Could you check a few things on this model? Use its own coordinates, in mm. A direction names the side the tool comes from. Coordinates: 2 decimals unless noted, no trailing zeros. Write each loop counter-clockwise with the first axis right and the second up, starting at its lowest first coordinate (ties: lowest second). Pieces come first, ordered by that corner, then holes. Notation, with made-up numbers: M 51,67.5 L 110,67.5 A14 cw 110,76.5 Z; hole C 2,17 d4. An arc over 180 degrees is marked long. Answer as CSV lines item,"result". Start each with the question number.
Item 1: Suppose I cut it at C-C, the plane y = -25. Write out the boundary of the cut face in (x, z), and give its area (3 significant figures).
Item 2: Suppose I cut it at B-B, the plane x = 7.62. Write out the boundary of the cut face in (y, z) (1 decimal).
Item 3: Suppose I cut it at A-A, the plane y = -29.21. Write out the boundary of the cut face in (x, z).
Item 4: If I drill on line 1 along Y through (x, z) = (7.62, 1.3) (1 decimal); line 2 along Y through (x, z) = (8.5, 2.35); line 3 along X through (y, z) = (-23, 1.9), over which ranges is the centre line in solid material (lowest first)? Write a range as [from, to].
Item 5: I'm going to push a flat-ended pin straight in: P1, Ø1.3, axis at y = -10, z = 1.5, coming from the -X side. Where does the tip first touch, or does it pass through?
Item 6: We'd pull the mould along Y, two halves only. Please class faces 1 (the flat face through (14, -5.08, 1)), 2 (the flat face through (8, -16, 0)), 3 (the cylindrical face through (7.67, -13.97, 1.25)): +Y half, -Y half, draft (parallel to the pull), parting line (faces both ways), or undercut.
Item 7: On a 3-axis mill with a long thin cutter (end or side, diameter ignored), from which of +Z, -Z, +X, -X, +Y, -Y can I reach the whole of each face in a straight line? I mean faces 4 (the flat face through (8, -33.02, 1)), 5 (the flat face through (13.018, -19, 1)), 6 (the flat face through (1, -5.08, 1)), 7 (the cylindrical face through (7.571, -6.986, 1.252)). Say none if no direction works.
Autodesk Inventor part; units mm, degrees
ref_plane "YZ Plane" through (0, 0, 0) normal (1, 0, 0) x (0, 1, 0)
ref_plane "XZ Plane" through (0, 0, 0) normal (0, 1, 0) x (-1, 0, 0)
ref_plane "XY Plane" through (0, 0, 0) normal (0, 0, 1) x (1, 0, 0)
sketch "Sketch1" plane through (0, 0, 0) normal (0, 0, 1) x (1, 0, 0)
  line L0 (0, 0) -> (15.24, 0)
  line L1 (15.24, 0) -> (15.24, -5.08)
  line L2 (15.24, -5.08) -> (13.0175, -5.08)
  line L3 (13.0175, -5.08) -> (13.0175, -33.02)
  line L4 (0, 0) -> (0, -5.08)
  line L5 (0, -5.08) -> (2.2225, -5.08)
  line L6 (2.2225, -5.08) -> (2.2225, -33.02)
  line L7 (2.2225, -33.02) -> (13.0175, -33.02)
  circle A0 centre (7.62, -29.21) radius 2.2225
  line L8 (7.62, -6.985) -> (7.62, -6.985)
  line L9 (9.8425, -9.2075) -> (9.8425, -11.7475)
  line L10 (7.62, -13.97) -> (7.62, -13.97)
  line L11 (5.3975, -11.7475) -> (5.3975, -9.2075)
  arc A1 (9.8425, -9.2075) -> (7.62, -6.985) centre (7.62, -9.2075) ccw
  arc A2 (7.62, -6.985) -> (5.3975, -9.2075) centre (7.62, -9.2075) ccw
  arc A3 (5.3975, -11.7475) -> (7.62, -13.97) centre (7.62, -11.7475) ccw
  arc A4 (7.62, -13.97) -> (9.8425, -11.7475) centre (7.62, -11.7475) ccw
  point P0 (9.8425, -13.97)
  point P1 (9.8425, -6.985)
  dimension "d0" = 15.24
  dimension "d1" = 5.08
  dimension "d2" = 2.2225
  dimension "d3" = 27.94
  dimension "d4" = 2.2225
  dimension "d5" = 4.445
  dimension "d6" = 3.81
  dimension "d7" = 6.985
  dimension "d8" = 6.985
  dimension "d9" = 2.2225
extrude "Extrusion1" add sketch "Sketch1" along normal blind 2.54
properties part number "MotorMount" material "Polycarbonate, Clear"
Ans:
1,outline,"M 2.22,0 L 13.02,0 L 13.02,2.54 L 2.22,2.54 Z"
1,area,"27.4 mm^2"
2,outline,"M -33,0 L -31.4,0 L -31.4,2.5 L -33,2.5 Z; M -27,0 L -14,0 L -14,2.5 L -27,2.5 Z; M -7,0 L 0,0 L 0,2.5 L -7,2.5 Z"
3,outline,"M 2.22,0 L 5.4,0 L 5.4,2.54 L 2.22,2.54 Z; M 9.84,0 L 13.02,0 L 13.02,2.54 L 9.84,2.54 Z"
4,line 1,"y = [-33, -31.4], [-27, -14], [-7, 0]"
4,line 2,"y = [-33.02, -31.25], [-27.17, -13.79], [-7.17, 0]"
4,line 3,"x = [2.22, 13.02]"
5,P1,"stops at x = 2.22"
6,face 1,"-Y half"
6,face 2,"draft"
6,face 3,"undercut"
7,face 4,"+Z, -Z, +X, -X, -Y"
7,face 5,"+Z, -Z, +X, -Y"
7,face 6,"+Z, -Z, -X, -Y"
7,face 7,"+Z, -Z"
